For this review, take the finished solid that the model builds, in its own axes (mm). Face numbers are marked on the shaded views. Give positions to 0.01 mm unless a question says otherwise; leave off trailing zeros. Write each loop counter-clockwise with the first axis right and the second up, starting at its lowest first coordinate (ties: lowest second). Pieces come first, ordered by that corner, then holes. Notation, with made-up numbers: (62.25, -24) -> (74.25, -24) arc R15 cw to (74.25, 2) -> close; hole circle Ø6 at (7, -39). An arc over 180 degrees is marked (long way). Write item = value, one per line.
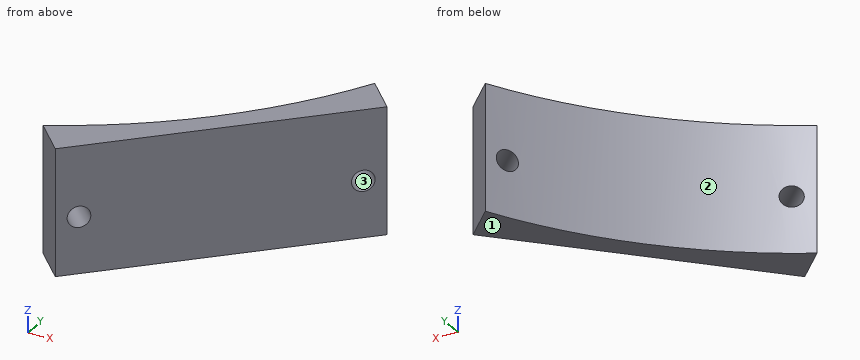
```python
from build123d import *

# Parameters (mm, degrees)
CYLINDER1768_R              = 1.5
CYLINDER1768_DEPTH          = 60
CYLINDER1765_R              = 1.5
CYLINDER1765_DEPTH          = 60
CYLINDER1766_R              = 1.5
CYLINDER1766_DEPTH          = 60
CYLINDER1767_R              = 1.5
CYLINDER1767_DEPTH          = 60
COMPOUND900_PLACEMENT_ANGLE = 225
CYLINDER1771_R              = 1.5
CYLINDER1771_DEPTH          = 50
COMPOUND903_PLACEMENT_ANGLE = 225
CYLINDER1770_R              = 1.5
CYLINDER1770_DEPTH          = 50
COMPOUND904_PLACEMENT_ANGLE = 225
CYLINDER1769_R              = 74
CYLINDER1769_DEPTH          = 40
BOX718_W                    = 42
BOX718_H                    = 10
BOX718_DEPTH                = 18
COMPOUND901_PLACEMENT_ANGLE = 225


with BuildPart() as obj1:
    # Cylinder1768 → Cylinder1768 (new body)
    with BuildSketch(Plane(origin=(-24, 73, -80), x_dir=(1, 0, 0), z_dir=(0, 0, 1))):
        Circle(CYLINDER1768_R)
    extrude(amount=CYLINDER1768_DEPTH)


with BuildPart() as obj2:
    # Cylinder1765 → Cylinder1765 (new body)
    with BuildSketch(Plane(origin=(-15, 135, -80), x_dir=(1, 0, 0), z_dir=(0, 0, 1))):
        Circle(CYLINDER1765_R)
    extrude(amount=CYLINDER1765_DEPTH)


with BuildPart() as obj3:
    # Cylinder1766 → Cylinder1766 (new body)
    with BuildSketch(Plane(origin=(15, 135, -80), x_dir=(1, 0, 0), z_dir=(0, 0, 1))):
        Circle(CYLINDER1766_R)
    extrude(amount=CYLINDER1766_DEPTH)


with BuildPart() as compound900:
    # Cylinder1767 → Cylinder1767 (new body)
    with BuildSketch(Plane(origin=(24, 73, -80), x_dir=(1, 0, 0), z_dir=(0, 0, 1))):
        Circle(CYLINDER1767_R)
    extrude(amount=CYLINDER1767_DEPTH)

    # Compound900: union obj1, obj2, obj3
    add(obj1.part)
    add(obj2.part)
    add(obj3.part)


with BuildPart() as compound900_1:
    # Compound900 placement: moved
    add(compound900.part.moved(Location((0, 0, 100))).rotate(Axis((0, 0, 100), (0, 0, 1)), COMPOUND900_PLACEMENT_ANGLE))


with BuildPart() as compound903:
    # Cylinder1771 → Cylinder1771 (new body)
    with BuildSketch(Plane(origin=(18, 100, 72), x_dir=(1, 0, 0), z_dir=(0, -1, 0))):
        Circle(CYLINDER1771_R)
    extrude(amount=CYLINDER1771_DEPTH)


with BuildPart() as compound903_1:
    # Compound903 placement: moved
    add(compound903.part.rotate(Axis((0, 0, 0), (0, 0, 1)), COMPOUND903_PLACEMENT_ANGLE))


with BuildPart() as compound902:
    # Cylinder1770 → Cylinder1770 (new body)
    with BuildSketch(Plane(origin=(-18, 100, 72), x_dir=(1, 0, 0), z_dir=(0, -1, 0))):
        Circle(CYLINDER1770_R)
    extrude(amount=CYLINDER1770_DEPTH)


with BuildPart() as compound902_1:
    # Compound904 placement: moved
    add(compound902.part.rotate(Axis((0, 0, 0), (0, 0, 1)), COMPOUND904_PLACEMENT_ANGLE))

    # Compound902: union Compound903
    add(compound903_1.part)


with BuildPart() as compound902_2:
    # Compound902 placement: moved
    add(compound902_1.part.moved(Location((0, 0, 1))))


with BuildPart() as obj4:
    # Cylinder1769 → Cylinder1769 (new body)
    with BuildSketch(Plane.XY.offset(44)):
        Circle(CYLINDER1769_R)
    extrude(amount=CYLINDER1769_DEPTH)


with BuildPart() as cut527:
    # Box718 → Box718 (new body)
    with BuildSketch(Plane(origin=(-21, -23, 22), x_dir=(1, 0, 0), z_dir=(0, 0, 1))):
        with Locations((21, 5)):
            Rectangle(BOX718_W, BOX718_H)
    extrude(amount=BOX718_DEPTH)


with BuildPart() as cut527_1:
    # Compound901 placement: moved
    add(cut527.part.moved(Location((63.64, -63.64, 43))).rotate(Axis((63.64, -63.64, 43), (0, 0, 1)), COMPOUND901_PLACEMENT_ANGLE))

    # Cut525: cut obj4
    add(obj4.part, mode=Mode.SUBTRACT)

    # Cut526: cut Compound902
    add(compound902_2.part, mode=Mode.SUBTRACT)

    # Cut527: cut Compound900
    add(compound900_1.part, mode=Mode.SUBTRACT)


solid = cut527_1.part
```
(1) The part is to be moulded in two halves that separate along X. For the marked faces 1, 2 and 3, say which applies: released by +X, released by -X, zero draft, split by the parting line, or undercut.
Answers below:
face_1 = zero draft
face_2 = released by -X
face_3 = undercut
(2) Take a section at A-A (z = 75). Write out the cut boundary in (x, y).
Answers below:
outline = (35.33, -65.02) -> (39.6, -69.3) -> (69.3, -39.6) -> (65.02, -35.33) arc R74 cw to start
(3) To check wall thickness, follow probe 1 along X at (y, z) = (-65, 73); probe 2 along Y at (x, z) = (45.5, 80.75); probe 3 along X at (y, z) = (-50, 66.25). State the ranges of each line that lie inside material, in increasing order.
Answers below:
probe_1 = 35.37 to 37.42, 41.67 to 43.9
probe_2 = -63.4 to -58.36
probe_3 = 54.55 to 58.9
(4) For pin 1 (1 mm diameter, centred on y = -39, z = 72, fed in from -X); pin 2 (6 mm diameter, centred on x = 52.5, y = -52, fed in from +Z); pin 3 (5 mm diameter, centred on y = -39, z = 80.5, fed in from -X); pin 4 (8 mm diameter, centred on x = 39.5, z = 74, fed in from -Y), all flat-tipped, find the tip position at first contact; note any pin that passes through.
Answers below:
pin_1 = 62.58
pin_2 = 83
pin_3 = 61.27
pin_4 = -69.3
(5) Take a section at B-B (y = -61.5). Write out the cut boundary in (x, z), plus the area to 3 significant figures.
Answers below:
outline = (41.16, 65) -> (47.4, 65) -> (47.4, 83) -> (41.16, 83) -> close
area = 112 mm^2
